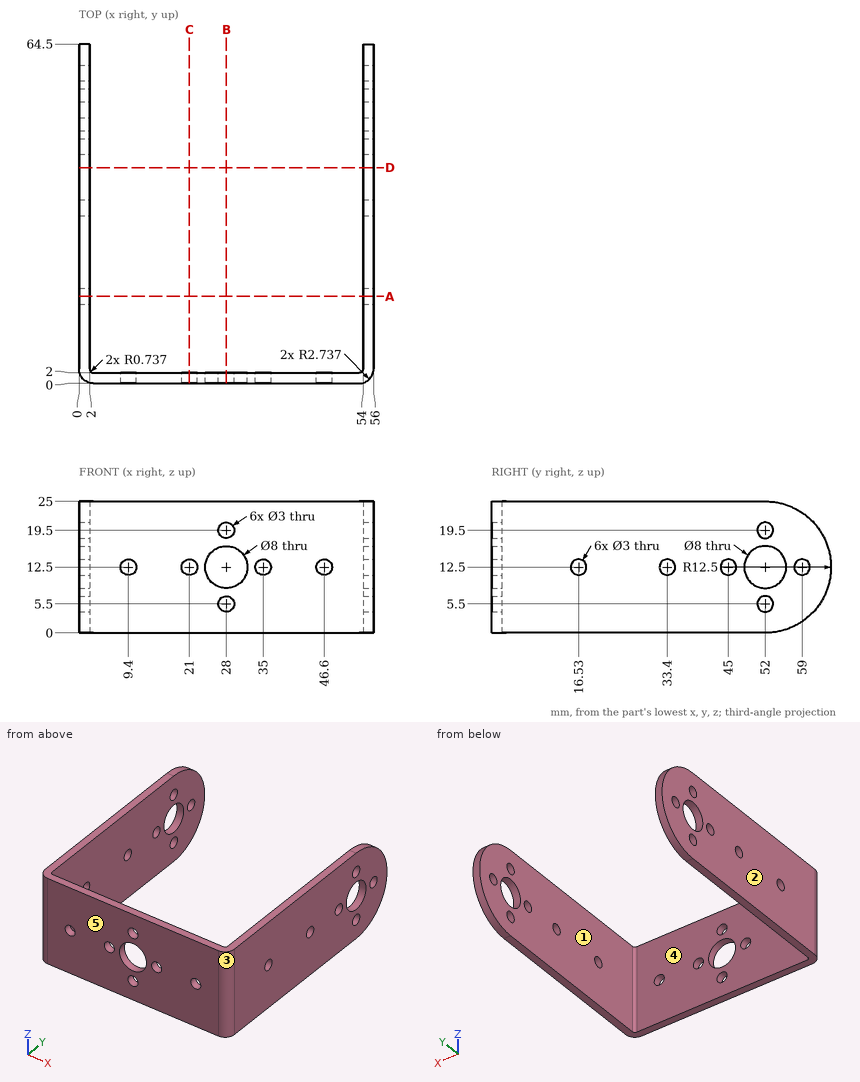
Print and shaded views of the part. All mm, measured from the part's lowest x, y and z. A direction names the side the tool comes from. Round coordinates to 2 decimals unless told otherwise and drop trailing zeros. Write each loop counter-clockwise with the first axis right and the second up, starting at its lowest first coordinate (ties: lowest second). Pieces come first, ordered by that corner, then holes. Notation, with made-up numbers: (-10, 37) -> (10, 37) arc R36 ccw to (10, 71) -> close; hole circle Ø8 at (-13, 79). An arc over 180 degrees is marked (long way). Return JSON: item names as keys, results as strings. Group by question number.
Q1. Mould opens along X. For the marked faces 1, 2 and 3 say: pulls with the +X half, pulls with the -X half, needs draft (parallel to the pull), parting line crosses it, or undercut.
Q2. Saw through at A-A on y = 16.53. Write the cut outline in (x, z).
Q3. Probe L1, parallel to Z at x = 28, y = 1.4; L2, parallel to X at y = 10, z = 2; L3, parallel to Y at x = 54.4, z = 12.5. List the from-to ranges inside material, lowest first. Write a range as [from, to].
Q4. Which spindle directions (+Z, -Z, +X, -X, +Y, -Y) get a long thin tool onto all of the face, cutting with end or side? Do the marked faces 4 and 5. Say none if no direction does.
Q5. Saw through at C-C on x = 21. Write the cut outline in (y, z).
Q6. Saw through at D-D on y = 41. Write the cut outline in (x, z), plus the area to 3 significant figures.
Q7. Saw through at B-B on x = 28. Write the cut outline in (y, z), plus the area to 3 significant figures.
Answer:
{
 "1": {"face 1": "undercut", "face 2": "pulls with the -X half", "face 3": "pulls with the +X half"},
 "2": {"outline": "(0, 0) -> (2, 0) -> (2, 11) -> (0, 11) -> close; (0, 14) -> (2, 14) -> (2, 25) -> (0, 25) -> close; (54, 0) -> (56, 0) -> (56, 11) -> (54, 11) -> close; (54, 14) -> (56, 14) -> (56, 25) -> (54, 25) -> close"},
 "3": {"L1": "[0, 4], [7, 8.5], [16.5, 18], [21, 25]", "L2": "[0, 2], [54, 56]", "L3": "[0.25, 15.03], [18.03, 31.9], [34.9, 43.5], [46.5, 48], [56, 57.5], [60.5, 64.5]"},
 "4": {"face 4": "+Z, -Z, +Y", "face 5": "+Z, -Z, +X, -X, -Y"},
 "5": {"outline": "(0, 0) -> (2, 0) -> (2, 11) -> (0, 11) -> close; (0, 14) -> (2, 14) -> (2, 25) -> (0, 25) -> close"},
 "6": {"outline": "(0, 0) -> (2, 0) -> (2, 25) -> (0, 25) -> close; (54, 0) -> (56, 0) -> (56, 25) -> (54, 25) -> close", "area": "100 mm2"},
 "7": {"outline": "(0, 0) -> (2, 0) -> (2, 4) -> (0, 4) -> close; (0, 7) -> (2, 7) -> (2, 8.5) -> (0, 8.5) -> close; (0, 16.5) -> (2, 16.5) -> (2, 18) -> (0, 18) -> close; (0, 21) -> (2, 21) -> (2, 25) -> (0, 25) -> close", "area": "22.0 mm2"}
}
